```python
from build123d import *

# Parameters (mm, degrees)
SKETCH_1_W             = 170
SKETCH_1_H             = 20
EXTRUDE_1_DEPTH        = 70
CUT_EXTRUDE_1_DEPTH    = 164
SKETCH_3_R             = 5
CUT_EXTRUDE_2_DEPTH    = 3
SKETCH_4_R             = 2.6
CUT_EXTRUDE_3_DEPTH    = 3
SKETCH_5_W             = 3.06
SKETCH_5_H             = 50
EXTRUDE_2_DEPTH        = 4
MIRROR_START           = 170
MIRROR_1_DEPTH         = 170
MIRROR_START_2         = 334
MIRROR_1_2_OUTLINE_R   = 5
MIRROR_1_2_DEPTH       = 6
MIRROR_START_3         = 340
MIRROR_1_3_OUTLINE_W   = 50
MIRROR_1_3_OUTLINE_H   = 6.12
MIRROR_1_3_DEPTH       = 4
MIRROR_START_4         = 337
MIRROR_1_4_OUTLINE_R   = 5
MIRROR_1_4_OUTLINE_R_2 = 2.6
MIRROR_1_4_DEPTH       = 3
SKETCH_6_W             = 4
SKETCH_6_H             = 6.12
CUT_EXTRUDE_4_DEPTH    = 200


# Read off the part's stored shape, not the designer's step: the mirror step
with BuildPart() as part:
    # Sketch 1 → Extrude 1 (new body)
    with BuildSketch(Plane(origin=(0, 0, 0), x_dir=(1, 0, 0), z_dir=(0, 1, 0))):
        with Locations((85, 10)):
            Rectangle(SKETCH_1_W, SKETCH_1_H)
    extrude(amount=EXTRUDE_1_DEPTH)

    # Sketch 2 → Cut-Extrude 1 (cut)
    with BuildSketch(Plane(origin=(170, 0, 0), x_dir=(0, 0, -1), z_dir=(1, 0, 0))):
        Polygon((0, 70), (0, 20), (20, 70), align=None)
    extrude(amount=-CUT_EXTRUDE_1_DEPTH, mode=Mode.SUBTRACT)

    # Sketch 3 → Cut-Extrude 2 (cut)
    with BuildSketch(Plane(origin=(6, 0, 0), x_dir=(0, 0, -1), z_dir=(1, 0, 0))):
        with Locations((10, 60)):
            Circle(SKETCH_3_R)
    extrude(amount=-CUT_EXTRUDE_2_DEPTH, mode=Mode.SUBTRACT)

    # Sketch 4 → Cut-Extrude 3 (cut)
    with BuildSketch(Plane(origin=(3, 0, 0), x_dir=(0, 0, -1), z_dir=(1, 0, 0))):
        with Locations((10, 60)):
            Circle(SKETCH_4_R)
    extrude(amount=-CUT_EXTRUDE_3_DEPTH, mode=Mode.SUBTRACT)

    # Sketch 5 → Extrude 2 (add)
    with BuildSketch(Plane.ZY):
        with Locations((-11.53, 25)):
            Rectangle(SKETCH_5_W, SKETCH_5_H)
        with Locations((-8.47, 25)):
            Rectangle(SKETCH_5_W, SKETCH_5_H)
    extrude(amount=EXTRUDE_2_DEPTH)

    # Mirror 1 outline → Mirror 1 (add)
    with BuildSketch(Plane.YZ.offset(MIRROR_START)):
        Polygon((20, 0), (0, 0), (0, -20), (70, -20), align=None)
    extrude(amount=MIRROR_1_DEPTH)

    # Mirror 1 2 outline → Mirror 1 2 (add)
    with BuildSketch(Plane.YZ.offset(MIRROR_START_2)):
        Polygon((70, 0), (20, 0), (70, -20), align=None)
        with Locations((60, -10)):
            Circle(MIRROR_1_2_OUTLINE_R, mode=Mode.SUBTRACT)
    extrude(amount=MIRROR_1_2_DEPTH)

    # Mirror 1 3 outline → Mirror 1 3 (add)
    with BuildSketch(Plane.YZ.offset(MIRROR_START_3)):
        with Locations((25, -10)):
            Rectangle(MIRROR_1_3_OUTLINE_W, MIRROR_1_3_OUTLINE_H)
    extrude(amount=MIRROR_1_3_DEPTH)

    # Mirror 1 4 outline → Mirror 1 4 (add)
    with BuildSketch(Plane.YZ.offset(MIRROR_START_4)):
        with Locations((60, -10)):
            Circle(MIRROR_1_4_OUTLINE_R)
        with Locations((60, -10)):
            Circle(MIRROR_1_4_OUTLINE_R_2, mode=Mode.SUBTRACT)
    extrude(amount=MIRROR_1_4_DEPTH)

    # Sketch 6 → Cut-Extrude 4 (cut)
    with BuildSketch(Plane.XZ):
        Polygon((170, 0), (0, 0), (0, -6.94), (0, -13.06), (0, -20), (170, -20), align=None)
        with Locations((-2, -10)):
            Rectangle(SKETCH_6_W, SKETCH_6_H)
    extrude(amount=-CUT_EXTRUDE_4_DEPTH, mode=Mode.SUBTRACT)


solid = part.part
```
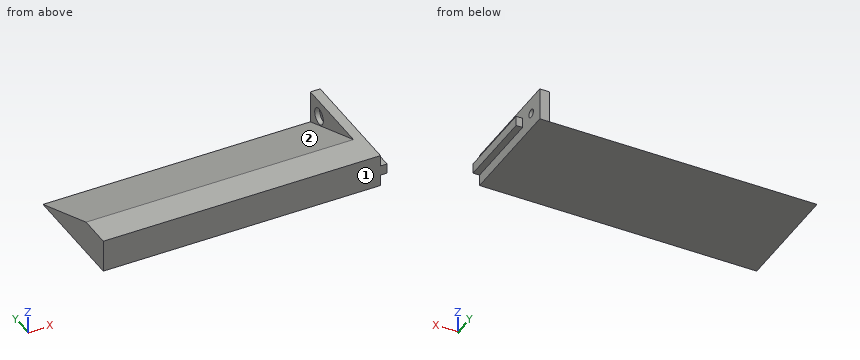
Design review of the part built by this model. Coordinates are the model's own, in mm. Face numbers are marked on the shaded views. A direction names the side the tool comes from. Coordinates: 2 decimals unless noted, no trailing zeros. Order: outer loops, then holes, each group sorted by start corner. A loop starts at its lowest first (then second) coordinate and runs counter-clockwise, first axis right, second up.
1) Take a section at B-B, the plane y = 60. Give the boundary of the cut face in (x, z), and give its area (3 significant figures).
2) Wall thickness on line 1 along Z through (x, y) = (335.65, 60); line 2 along X through (y, z) = (34, -2.75); line 3 along Z through (x, y) = (230.5, 38.5): over which ranges is each line inside the solid? List them lowest first.
3) Take a section at C-C, the plane z = -2.5. Give the boundary of the cut face in (x, y).
4) For the marked faces 1 and 2, list the 3-axis set-ups (+Z, -Z, +X, -X, +Y, -Y) from which the entire face can be reached by the end or side of a thin tool; tool diameter is ignored.
5) Take a section at A-A, the plane z = -10. Give the boundary of the cut face in (x, y), and give its area (3 significant figures).
6) Clearance check with flat-ended pins moving along their axes: pin 1 (10 mm diameter, centred on y = 62.5, z = -9, fed in from -X); pin 2 (3 mm diameter, centred on x = 342.5, y = 33.5, fed in from +Z); pin 3 (11.5 mm diameter, centred on y = 60, z = -10, fed in from +X); pin 4 (12 mm diameter, centred on x = 196.5, z = -3, fed in from -Y). State where each tip first meets the part, or that it passes through.
7) Take a section at D-D, the plane x = 310. Give the boundary of the cut face in (y, z), and give its area (3 significant figures).
Returned:
1. outline: (170, -20) - (340, -20) - (340, -12.6) - (337, -12.6) - (337, -15) - (334, -15) - (334, -16) - (170, -16) - close; (334, -5) - (337, -5) - (337, -7.4) - (340, -7.4) - (340, 0) - (334, 0) - close
1. area: 730 mm2
2. line 1: z = -20 to -15, -5 to 0
2. line 2: x = 334 to 340
2. line 3: z = -20 to -7.4
3. outline: (170, 0) - (340, 0) - (340, 70) - (334, 70) - (334, 26.25) - (170, 26.25) - close
4. face 1: +Z, -Z, +X, -X, -Y
4. face 2: +Z, -X, +Y
5. outline: (170, 0) - (344, 0) - (344, 50) - (340, 50) - (340, 57.4) - (337, 57.4) - (337, 55) - (334, 55) - (334, 45) - (170, 45) - close; (334, 65) - (337, 65) - (337, 62.6) - (340, 62.6) - (340, 70) - (334, 70) - close
5. area: 7,950 mm2
6. pin 1: stops at x = 334
6. pin 2: stops at z = -6.94
6. pin 3: stops at x = 340
6. pin 4: stops at y = 0
7. outline: (0, -20) - (70, -20) - (20, 0) - (0, 0) - close
7. area: 900 mm2
